The listing builds one solid part. Answer for the finished solid, in the listing's coordinates (mm). Face numbers are marked on the shaded views. A direction names the side the tool comes from. Coordinates: 2 decimals unless noted, no trailing zeros. Order: outer loops, then holes, each group sorted by start corner. A loop starts at its lowest first (then second) coordinate and runs counter-clockwise, first axis right, second up. Notation, with made-up numbers: (20.25, 40) -> (56.25, 40) arc R20 cw to (56.25, 55) -> close; hole circle Ø6 at (-20, 24). An arc over 180 degrees is marked (long way). Write each question's results on one line, items separated by ' | '. Start each with the question number.
(1) The part is cut by section C-C, the plane x = 0. Give the vertices of the cut face in (y, z), then the cut area to 3 significant figures.
(2) A tool of negligible diameter and unlimited length cuts with its end or side. For the marked faces 1 and 2, from which of +Z, -Z, +X, -X, +Y, -Y can it reach the whole face along a straight path? Write none if from no direction.
(3) Given pin 1 (3.5 mm diameter, centred on y = -5, z = 4.5, fed in from -X); pin 2 (5 mm diameter, centred on x = 0.5, z = 10, fed in from +Y), each flat-ended and moving along its own axis, determine where each tip first touches the part or whether it passes through.
(4) The part is cut by section B-B, the plane z = 3. Give the vertices of the cut face in (x, y).
(5) Straight lines are drawn through the part: L1, parallel to Z at x = 9.25, y = -5.75; L2, parallel to X at y = -6, z = 11.25; L3, parallel to X at y = -20, z = 9. For each, find the intervals that lie inside material, in ascending order.
(6) The part is cut by section D-D, the plane y = -20.75. Give the vertices of the cut face in (x, z), then the cut area to 3 significant figures.
(7) Determine the mould class of the marked faces 3, 4 and 5 for opening direction X: +X half, -X half, draft (parallel to the pull), parting line (faces both ways), or undercut.
(8) The part is cut by section A-A, the plane y = -13.5. Give the vertices of the cut face in (x, z).
```python
from build123d import *

# Parameters (mm, degrees)
BOSS_EXTRU_1_DEPTH      = 11.5
ENL_V_MAT_EXTRU_1_REACH = 34.715
ESQUISSE3_R             = 4.5
CONG_1_R                = 5.75


with BuildPart() as part:
    # Esquisse1 → Boss.-Extru.1 (new body)
    with BuildSketch(Plane.XY):
        with BuildLine():
            Line((-10, 0), (-8.5, 0))
            Line((-8.5, 0), (-8.5, -18.5))
            ThreePointArc((-8.5, -18.5), (0, -21.195436549), (8.5, -18.5))
            Line((8.5, -18.5), (8.5, 0))
            Line((8.5, 0), (10, 0))
            Line((10, 0), (10, -19.882791199))
            ThreePointArc((10, -19.882791199), (0, -23.195436549), (-10, -19.882791199))
            Line((-10, -19.882791199), (-10, 0))
        make_face()
    extrude(amount=BOSS_EXTRU_1_DEPTH)

    # Enlèv. mat.-Extru.1: up to this face of the body (flat: up to its plane)
    enl_v_mat_extru_1_end = Plane(part.part.faces().sort_by_distance((-10, -9.9413956, 5.75))[0])
    # Esquisse3 → Enlèv. mat.-Extru.1 (cut, up to the picked face)
    with BuildSketch(Plane(origin=(10, 0, 0), x_dir=(0, 0, -1), z_dir=(1, 0, 0)), mode=Mode.PRIVATE) as enl_v_mat_extru_1_sk1:
        with Locations(Location((-5.75, -5.75, 0), (0, 0, 90))):
            Circle(ESQUISSE3_R)
    enl_v_mat_extru_1_tool1 = split(extrude(enl_v_mat_extru_1_sk1.sketch, amount=-ENL_V_MAT_EXTRU_1_REACH, mode=Mode.PRIVATE), bisect_by=enl_v_mat_extru_1_end, keep=Keep.BOTH, mode=Mode.PRIVATE)
    add(enl_v_mat_extru_1_tool1.solids().sort_by(Axis((10, -5.75, 5.75), (-1, 0, 0)))[0], mode=Mode.SUBTRACT)

    # Congé1
    cong_1_edges = [part.edges().sort_by_distance(p)[0] for p in [
        (-9.25, 0, 0),
        (-9.25, 0, 11.5),
        (9.25, 0, 0),
        (9.25, 0, 11.5),
    ]]
    fillet(cong_1_edges, radius=CONG_1_R - 0.0001)  # a hair under: the kernel refuses the full size


solid = part.part
```
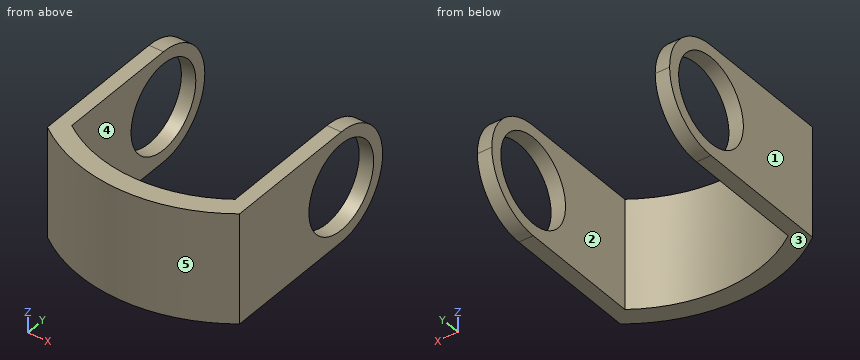
Established:
1) outline: (-23.2, 0) -> (-21.2, 0) -> (-21.2, 11.5) -> (-23.2, 11.5) -> close | area: 23.0 mm^2
2) face 1: +Z, -Z, -X, +Y, -Y | face 2: +Z, -Z, +Y
3) pin 1: passes through | pin 2: stops at y = -20.89
4) outline: (-10, -19.88) arc R16.75 ccw to (10, -19.88) -> (10, -9.31) -> (8.5, -9.31) -> (8.5, -18.5) arc R14.75 cw to (-8.5, -18.5) -> (-8.5, -9.31) -> (-10, -9.31) -> close; (-10, -2.19) -> (-8.5, -2.19) -> (-8.5, -0.7) -> (-10, -0.7) -> close; (8.5, -2.19) -> (10, -2.19) -> (10, -0.7) -> (8.5, -0.7) -> close
5) L1: z = 0 to 1.25, 10.25 to 11.5 | L2: x = -10 to -8.5, 8.5 to 10 | L3: x = -9.84 to -5.82, 5.82 to 9.84
6) outline: (-8.71, 0) -> (-3.6, 0) -> (-3.6, 11.5) -> (-8.71, 11.5) -> close; (3.6, 0) -> (8.71, 0) -> (8.71, 11.5) -> (3.6, 11.5) -> close | area: 118 mm^2
7) face 3: draft | face 4: undercut | face 5: parting line
8) outline: (-10, 0) -> (-8.5, 0) -> (-8.5, 11.5) -> (-10, 11.5) -> close; (8.5, 0) -> (10, 0) -> (10, 11.5) -> (8.5, 11.5) -> close
